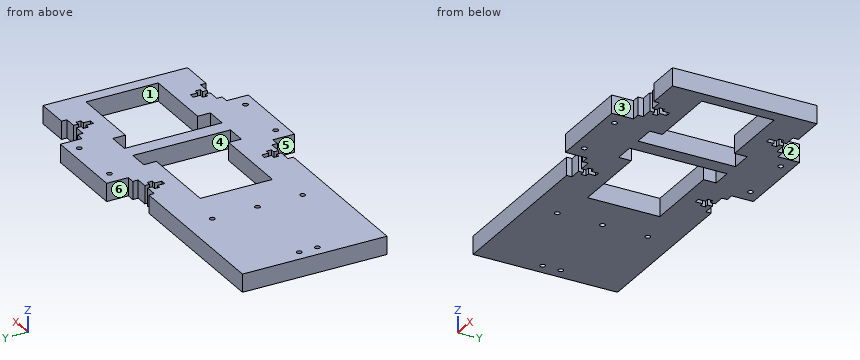
```python
from build123d import *

# Parameters (mm, degrees)
SKETCH1_R           = 1.42
BOSS_EXTRUDE1_DEPTH = 10


with BuildPart() as part:
    # Sketch1 → Boss-Extrude1 (new body)
    with BuildSketch(Plane.XY):
        Polygon((109, 80), (109, 77), (115.58, 77), (115.58, 74.4), (113.33, 74.4), (113.33, 71.6), (115.58, 71.6), (115.58, 67.6), (118.42, 67.6), (118.42, 71.6), (120.67, 71.6), (120.67, 74.4), (118.42, 74.4), (118.42, 77), (125, 77), (125, 80), (143.417515172, 80), (143.417515172, 60), (143.417515172, 20), (143.417515172, 0), (125, 0), (125, 3), (118.42, 3), (118.42, 5.6), (120.67, 5.6), (120.67, 8.4), (118.42, 8.4), (118.42, 12.4), (115.58, 12.4), (115.58, 8.4), (113.33, 8.4), (113.33, 5.6), (115.58, 5.6), (115.58, 3), (109, 3), (109, 0), (104.593570259, 0), (104.593570259, -12), (58.593570259, -12), (58.593570259, 0), (54.187140517, 0), (54.187140517, 3), (47.607140517, 3), (47.607140517, 5.6), (49.857140517, 5.6), (49.857140517, 8.4), (47.607140517, 8.4), (47.607140517, 12.4), (44.767140517, 12.4), (44.767140517, 8.4), (42.517140517, 8.4), (42.517140517, 5.6), (44.767140517, 5.6), (44.767140517, 3), (38.187140517, 3), (38.187140517, 0), (0, 0), (-15.602079829, 0), (-54.853791786, 0), (-54.853791786, 80), (-15.602079829, 80), (5, 80), (38.187140517, 80), (38.187140517, 77), (44.767140517, 77), (44.767140517, 74.4), (42.517140517, 74.4), (42.517140517, 71.6), (44.767140517, 71.6), (44.767140517, 67.6), (47.607140517, 67.6), (47.607140517, 71.6), (49.857140517, 71.6), (49.857140517, 74.4), (47.607140517, 74.4), (47.607140517, 77), (54.187140517, 77), (54.187140517, 80), (58.593570259, 80), (58.593570259, 92), (104.593570259, 92), (104.593570259, 80), align=None)
        with Locations((2.037759908, 40)):
            Circle(SKETCH1_R, mode=Mode.SUBTRACT)
        with Locations((2.037759908, 65)):
            Circle(SKETCH1_R, mode=Mode.SUBTRACT)
        with Locations((2.037759908, 15)):
            Circle(SKETCH1_R, mode=Mode.SUBTRACT)
        with Locations((66.593570259, 86)):
            Circle(SKETCH1_R, mode=Mode.SUBTRACT)
        with Locations((96.593570259, 86)):
            Circle(SKETCH1_R, mode=Mode.SUBTRACT)
        with Locations((96.593570259, -6)):
            Circle(SKETCH1_R, mode=Mode.SUBTRACT)
        with Locations((66.593570259, -6)):
            Circle(SKETCH1_R, mode=Mode.SUBTRACT)
        with Locations((-48.502415741, 45)):
            Circle(SKETCH1_R, mode=Mode.SUBTRACT)
        with Locations((-48.502415741, 35)):
            Circle(SKETCH1_R, mode=Mode.SUBTRACT)
        Polygon((136.600558962, 60), (136.600558962, 20), (97.442765105, 20), (97.442765105, 13), (85.759642836, 13), (85.759642836, 67), (97.442765105, 67), (97.442765105, 60), align=None, mode=Mode.SUBTRACT)
        Polygon((23.079003763, 60), (66.593570259, 60), (66.593570259, 67), (77.427497681, 67), (77.427497681, 13), (66.593570259, 13), (66.593570259, 20), (23.079003763, 20), align=None, mode=Mode.SUBTRACT)
    extrude(amount=BOSS_EXTRUDE1_DEPTH)


solid = part.part
```
Check sheet for the modelled part. Datum: model origin and axes. Units: mm. Face numbers are marked on the shaded views. A direction names the side the tool comes from. Coordinates: 2 decimals unless noted, no trailing zeros. Loops run counter-clockwise (first coordinate to the right, second up) from the corner with the lowest first, then second, coordinate; pieces in that order, holes last. Notation, with made-up numbers: M -37.75,-9 L -24.75,-9 A33 cw -24.75,29 Z; hole C 6,59 d11. An arc over 180 degrees is marked long. Answer as a JSON object with one key per item and string values.
1. Sectioned sample at B-B on z = 5.5. Count the separate pieces of the cut face and the enclosed holes in it, and give its area (3 significant figures).
Outcome:
{"separate pieces": "1", "enclosed holes": "11", "area": "12,000 mm²"}
2. Scan lines: L1, parallel to X at y = 70.5, z = 7; L2, parallel to X at y = 38.5, z = 6; L3, parallel to Y at x = 120, z = 1. Record each from-to range of solid material in increasing order. Write a range as from..to.
Outcome:
{"L1": "-54.85..44.77, 47.61..115.58, 118.42..143.42", "L2": "-54.85..23.08, 77.43..85.76, 136.6..143.42", "L3": "3..5.6, 8.4..20, 60..71.6, 74.4..77"}
3. Sectioned sample at A-A on x = 40. Record the cut outline in (y, z), and give its area (3 significant figures).
Outcome:
{"outline": "M 3,0 L 20,0 L 20,10 L 3,10 Z; M 60,0 L 77,0 L 77,10 L 60,10 Z", "area": "340 mm²"}
4. Depth check by flat-ended pin: P1, Ø2, axis at x = 51.5, z = 6.5, coming from the +Y side; P2, Ø5, axis at y = 83.5, z = 4.5, coming from the +X side; P3, Ø2.5, axis at x = 2.04, y = 65, coming from the +Z side; P4, Ø0.7, axis at x = 119, z = 4, coming from the -Y side. Enter the tip coordinate at first touch or a pass-through.
Outcome:
{"P1": "y = 77", "P2": "x = 104.59", "P3": "through", "P4": "y = 3"}
5. Release check for a two-part mould opening along Y. For the marked faces 1 and 2 record: pulls with the +Y half, pulls with the -Y half, needs draft (parallel to the pull), parting line crosses it, or undercut.
Outcome:
{"face 1": "undercut", "face 2": "needs draft"}
6. Access from +Z, -Z, +X, -X, +Y, -Y to the whole of each face (thin tool, end or side, straight path). Record for the marked faces 3, 4, 5 and 6.
Outcome:
{"face 3": "+Z, -Z, +X, -Y", "face 4": "+Z, -Z", "face 5": "+Z, -Z, -X, -Y", "face 6": "+Z, -Z, -X, +Y"}
